Input: part model. Units: mm. Frame: model coordinates. Round coordinates to 2 decimals unless told otherwise and drop trailing zeros. Order: outer loops, then holes, each group sorted by start corner. A loop starts at its lowest first (then second) coordinate and runs counter-clockwise, first axis right, second up.
Item 1: Line query: L1, parallel to Y at x = -10.25, z = -2.75; L2, parallel to X at y = 77.5, z = -7.75; L3, parallel to Z at x = 1.75, y = 80.25. Output: solid intervals per line, ascending.
Item 2: Cut plane B-B on x = -8.5. Output: boundary loops of the cut face in (y, z).
Item 3: First-contact query: pin 1 (2 mm diameter, centred on x = -1, y = 77, fed in from +Z); pin 2 (6 mm diameter, centred on x = 8.5, z = -12.5, fed in from +Y); pin 3 (8 mm diameter, centred on y = 88, z = -3.5, fed in from -X); pin 4 (5 mm diameter, centred on x = 0, y = 89.5, fed in from -Z). Flat tips, straight axial feed; report the tip coordinate or a pass-through.
Item 4: Cut plane A-A on x = 7.5. Output: boundary loops of the cut face in (y, z).
```python
from build123d import *

# Parameters (mm, degrees)
SKETCH2_R           = 12.2
BOSS_EXTRUDE1_DEPTH = 15
BOSS_EXTRUDE2_DEPTH = 25


with BuildPart() as part:
    # Sketch2 → Boss-Extrude1 (new body)
    with BuildSketch(Plane(origin=(0, 2.526178565, -14.326670571), x_dir=(0, -0.984807753, -0.173648178), z_dir=(0, -0.173648178, 0.984807753))):
        with Locations((-84.490615604, 0)):
            Circle(SKETCH2_R)
    extrude(amount=-BOSS_EXTRUDE1_DEPTH)


with BuildPart() as body_2:
    # Sketch1 → Boss-Extrude2 (new body, symmetric)
    with BuildSketch(Plane(origin=(0, 0, 0), x_dir=(0, 0, -1), z_dir=(1, 0, 0))):
        with BuildLine():
            Line((4.367840897, 87.799360654), (2.460560139, 98.616087344))
            Line((2.460560139, 98.616087344), (1.59231925, 103.540126109))
            Line((1.59231925, 103.540126109), (11.44039678, 105.276607886))
            Line((11.44039678, 105.276607886), (16.545653204, 76.323259947))
            ThreePointArc((16.545653204, 76.323259947), (8.553554718, 80.041746373), (4.367840897, 87.799360654))
        make_face()
    extrude(amount=BOSS_EXTRUDE2_DEPTH, both=True)


with BuildPart() as part_1:
    add(part.part)

    # Combine1: cut body 2
    add(body_2.part, mode=Mode.SUBTRACT)


solid = part_1.part
```
From the geometry:
1. L1: y = 79.56 to 93
1. L2: x = -7.64 to 7.64
1. L3: z = -8.34 to -0.62
2. outline: (77.11, -1.17) - (78.71, -10.2) arc R14 cw to (87.8, -4.37) - (95.22, -3.06) - (94.35, 1.86) - close
3. pin 1: stops at z = -1.02
3. pin 2: stops at y = 79.23
3. pin 3: stops at x = -12.2
3. pin 4: stops at z = -4.53
4. outline: (76.26, -1.33) - (78.02, -11.31) arc R14 cw to (87.8, -4.37) - (96.08, -2.91) - (95.21, 2.02) - close
